Here's how the part is built. I have some questions about the finished solid (model axes, mm). Face numbers are marked on the shaded views. A direction names the side the tool comes from. Round coordinates to 2 decimals unless told otherwise and drop trailing zeros. Loops run counter-clockwise (first coordinate to the right, second up) from the corner with the lowest first, then second, coordinate; pieces in that order, holes last. Notation, with made-up numbers: M 4,64 L 48,64 A35 cw 48,102 Z; hole C -19.5,-5 d6. An arc over 180 degrees is marked long. Answer as CSV lines item,"result".
```python
from build123d import *

# Parameters (mm, degrees)
F0_R     = 32.5
F0_R_2   = 27.78
F1_DEPTH = 10
F0_R_3   = 1.6
F0_R_4   = 20.03
F2_DEPTH = 5


with BuildPart() as f1:
    # F0 (on Top) → F1 (new body)
    with BuildSketch(Plane.XY):
        Circle(F0_R)
        Circle(F0_R_2, mode=Mode.SUBTRACT)
    extrude(amount=F1_DEPTH)

    # F0 (on Top) → F2 (join)
    with BuildSketch(Plane.XY):
        Circle(F0_R_2)
        with Locations((0, -23.905)):
            Circle(F0_R_3, mode=Mode.SUBTRACT)
        with Locations((-23.905, 0)):
            Circle(F0_R_3, mode=Mode.SUBTRACT)
        Circle(F0_R_4, mode=Mode.SUBTRACT)
        with Locations((23.905, 0)):
            Circle(F0_R_3, mode=Mode.SUBTRACT)
        with Locations((0, 23.905)):
            Circle(F0_R_3, mode=Mode.SUBTRACT)
    extrude(amount=F2_DEPTH)


solid = f1.part
```
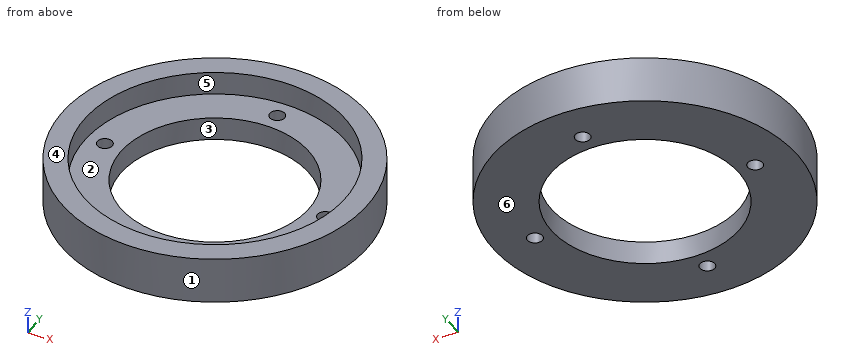
1. For P1, Ø10, axis at x = 13.5, y = -15.5, coming from the +Z side; P2, Ø2.5, axis at x = -23.905, y = 0, coming from the -Z side; P3, Ø5, axis at x = -6.5, z = 5, coming from the -Y side; P4, Ø2, axis at x = 4, z = 6, coming from the -Y side, each with a flat end and sliding along its axis, tell me the tip position at first contact or that it passes through.
Evaluation:
P1,"stops at z = 5"
P2,"passes through"
P3,"stops at y = -32.25"
P4,"stops at y = -32.36"
2. I want a section at B-B, the plane x = -10. Please give me the cut outline in (y, z).
Evaluation:
outline,"M -30.92,0 L -17.36,0 L -17.36,5 L -25.92,5 L -25.92,10 L -30.92,10 Z; M 17.36,0 L 30.92,0 L 30.92,10 L 25.92,10 L 25.92,5 L 17.36,5 Z"
3. Which directions (+Z, -Z, +X, -X, +Y, -Y) give clear straight access to the entire face, cutting with the end or side of a thin tool? Please do the marked faces 5 and 6.
Evaluation:
face 5,"+Z"
face 6,"-Z, +X, -X, +Y, -Y"
4. If I drill on line 1 (Z direction, x = -5.5, y = 23.5); line 2 (Y direction, x = -3, z = 5.5); line 3 (X direction, y = 3.5, z = 9.5), over which ranges is the centre line in solid material (lowest first)? Write a range as [from, to].
Evaluation:
line 1,"z = [0, 5]"
line 2,"y = [-32.36, -27.62], [27.62, 32.36]"
line 3,"x = [-32.31, -27.56], [27.56, 32.31]"
5. I want a section at D-D, the plane y = 7. Please give me the cut outline in (x, z), and give its area (3 significant figures).
Evaluation:
outline,"M -31.74,0 L -18.77,0 L -18.77,5 L -26.88,5 L -26.88,10 L -31.74,10 Z; M 18.77,0 L 31.74,0 L 31.74,10 L 26.88,10 L 26.88,5 L 18.77,5 Z"
area,"178 mm²"
6. I want a section at A-A, the plane y = 0. Please give me the cut outline in (x, z) (3 decimals), and give its area (3 significant figures).
Evaluation:
outline,"M -32.5,0 L -25.505,0 L -25.505,5 L -27.78,5 L -27.78,10 L -32.5,10 Z; M -22.305,0 L -20.03,0 L -20.03,5 L -22.305,5 Z; M 20.03,0 L 22.305,0 L 22.305,5 L 20.03,5 Z; M 25.505,0 L 32.5,0 L 32.5,10 L 27.78,10 L 27.78,5 L 25.505,5 Z"
area,"140 mm²"
7. We'd pull the mould along Y, two halves only. Please class the marked faces 1, 2, 3 and 4: pulls with the +Y half, pulls with the -Y half, needs draft (parallel to the pull), parting line crosses it, or undercut.
Evaluation:
face 1,"parting line crosses it"
face 2,"undercut"
face 3,"undercut"
face 4,"needs draft"
